```python
from build123d import *

# Parameters (mm, degrees)
SKETCH_1_W             = 36.9
SKETCH_1_H             = 36.9
EXTRUDE_1_DEPTH        = 20
SKETCH_2_R             = 4
CUT_EXTRUDE_1_DEPTH    = 36.9
SKETCH_3_R             = 6.5
CUT_EXTRUDE_2_DEPTH    = 3.5
CUT_EXTRUDE_3_DEPTH    = 51
FILLET_1_R             = 10
FILLET_2_R             = 5
SKETCH_5_W             = 16.9
SKETCH_5_H             = 16.9
SKETCH_5_W_2           = 7
SKETCH_5_H_2           = 7
CUT_EXTRUDE_4_DEPTH    = 16.55
HOLE_WIZARD_M3_1_D     = 2.5
HOLE_WIZARD_M3_1_DEPTH = 10
HOLE_WIZARD_M3_2_D     = 2.5
HOLE_WIZARD_M3_3_D     = 2.5
HOLE_WIZARD_M3_3_DEPTH = 10
FILLET_3_R             = 2
FILLET_7_R             = 2
CHAMFER_1_SIZE         = 0.3


with BuildPart() as part:
    # 草图1 → 凸台-拉伸1 (new, symmetric)
    with BuildSketch(Plane.XY):
        Rectangle(SKETCH_1_W, SKETCH_1_H)
    extrude(amount=EXTRUDE_1_DEPTH, both=True)

    # 草图2 → 切除-拉伸1 (cut)
    with BuildSketch(Plane(origin=(18.45, 0, 0), x_dir=(0, 0, -1), z_dir=(1, 0, 0))):
        with Locations((-11.25, -10)):
            Circle(SKETCH_2_R)
        Polygon((-1.5, 18.5), (-20, 0), (-20, 18.5), align=None)
    extrude(amount=-CUT_EXTRUDE_1_DEPTH, mode=Mode.SUBTRACT)

    # 草图3 → 切除-拉伸2 (cut)
    with BuildSketch(Plane(origin=(18.45, 0, 0), x_dir=(0, 0, -1), z_dir=(1, 0, 0))):
        with Locations((-11.25, -10)):
            Circle(SKETCH_3_R)
    cut_extrude_2 = extrude(amount=-CUT_EXTRUDE_2_DEPTH, mode=Mode.SUBTRACT)

    # 镜向1: 切除-拉伸2 across plane
    add(cut_extrude_2.mirror(Plane(origin=(0, 0, 0), x_dir=(0, 0, 1), z_dir=(1, 0, 0))), mode=Mode.SUBTRACT)

    # 草图4 → 切除-拉伸3 (cut)
    with BuildSketch(Plane(origin=(18.45, 0, 0), x_dir=(0, 0, -1), z_dir=(1, 0, 0))):
        Polygon((-20, 0), (-1.55, 0), (-1.55, 18.45), align=None)
    extrude(amount=-CUT_EXTRUDE_3_DEPTH, mode=Mode.SUBTRACT)

    # 圆角1
    fillet_1_edges = [part.edges().sort_by_distance(p)[0] for p in [
        (0, 0, 1.55),
    ]]
    fillet(fillet_1_edges, radius=FILLET_1_R)

    # 圆角2
    fillet_2_edges = [part.edges().sort_by_distance(p)[0] for p in [
        (0, -18.45, 20),
        (0, 0, 20),
    ]]
    fillet(fillet_2_edges, radius=FILLET_2_R)

    # 草图5 → 切除-拉伸4 (cut)
    with BuildSketch(Plane(origin=(0, 0, -20), x_dir=(-1, 0, 0), z_dir=(0, 0, -1))):
        Rectangle(SKETCH_5_W, SKETCH_5_H)
        with Locations((-11.95, 0)):
            Rectangle(SKETCH_5_W_2, SKETCH_5_H)
        with Locations((0, 11.95)):
            Rectangle(SKETCH_5_W, SKETCH_5_H_2)
        with Locations((11.95, 0)):
            Rectangle(SKETCH_5_W_2, SKETCH_5_H)
        with Locations((0, -11.95)):
            Rectangle(SKETCH_5_W, SKETCH_5_H_2)
    extrude(amount=-CUT_EXTRUDE_4_DEPTH, mode=Mode.SUBTRACT)

    # M3 螺纹孔1
    with Locations(Plane(origin=(0, 18.45, 0), x_dir=(1, 0, 0), z_dir=(0, 1, 0))):
        with Locations((-13.45, 10), (13.45, 10)):
            Hole(HOLE_WIZARD_M3_1_D / 2, depth=HOLE_WIZARD_M3_1_DEPTH)

    # M3 螺纹孔2 (through all)
    with Locations(Plane(origin=(18.45, 0, 0), x_dir=(0, 0, -1), z_dir=(1, 0, 0))):
        with Locations((10, -13.45)):
            hole_wizard_m3_2 = Hole(HOLE_WIZARD_M3_2_D / 2)

    # 镜向2: M3 螺纹孔2 across plane
    add(hole_wizard_m3_2.mirror(Plane(origin=(0, 0, 0), x_dir=(0, 0, 1), z_dir=(1, 0, 0))), mode=Mode.SUBTRACT)

    # M3 螺纹孔3
    with Locations(Plane(origin=(0, -18.45, 0), x_dir=(-1, 0, 0), z_dir=(0, -1, 0))):
        with Locations((10, 5), (-10, 5)):
            Hole(HOLE_WIZARD_M3_3_D / 2, depth=HOLE_WIZARD_M3_3_DEPTH)

    # 圆角3
    # the kernel refuses this fillet: 2 mm, written as the material it adds along each edge
    with BuildSketch(Plane(origin=(-15.45, 8.45, -20), x_dir=(1, 0, 0), z_dir=(0, 0, 1))) as fillet_3_piece_1_section:
        with BuildLine():
            CenterArc((FILLET_3_R, -FILLET_3_R), FILLET_3_R, 90, 90)
            Line((0, -FILLET_3_R), (0, 0))
            Line((0, 0), (FILLET_3_R, 0))
        make_face()
    fillet_3_piece_1 = extrude(amount=21.55, mode=Mode.PRIVATE)
    fillet_3_piece_1 = fillet_3_piece_1 - Plane(origin=(-13.45, 7.989094357, -10), x_dir=(-1, 0, 0), z_dir=(0, -1, 0)) * Cylinder(1.25, 52, mode=Mode.PRIVATE)
    add(fillet_3_piece_1)
    with BuildSketch(Plane(origin=(-15.45, -8.45, -20), x_dir=(0, 1, 0), z_dir=(0, 0, 1)), Plane(origin=(15.45, -8.45, -20), x_dir=(-1, 0, 0), z_dir=(0, 0, 1)), Plane(origin=(8.45, 15.45, -20), x_dir=(0, -1, 0), z_dir=(0, 0, 1)), Plane(origin=(-8.45, 15.45, -20), x_dir=(1, 0, 0), z_dir=(0, 0, 1))) as fillet_3_piece_2:
        with BuildLine():
            CenterArc((FILLET_3_R, -FILLET_3_R), FILLET_3_R, 90, 90)
            Line((0, -FILLET_3_R), (0, 0))
            Line((0, 0), (FILLET_3_R, 0))
        make_face()
    extrude(amount=21.55)
    with BuildSketch(Plane(origin=(-8.45, -15.45, -20), x_dir=(0, 1, 0), z_dir=(0, 0, 1))) as fillet_3_piece_3_section:
        with BuildLine():
            CenterArc((FILLET_3_R, -FILLET_3_R), FILLET_3_R, 90, 90)
            Line((0, -FILLET_3_R), (0, 0))
            Line((0, 0), (FILLET_3_R, 0))
        make_face()
    fillet_3_piece_3 = extrude(amount=21.55, mode=Mode.PRIVATE)
    fillet_3_piece_3 = fillet_3_piece_3 - Plane(origin=(-7.989094431, -13.45, -10), x_dir=(0, 0, 1), z_dir=(-1, 0, 0)) * Cylinder(1.25, 52, mode=Mode.PRIVATE)
    add(fillet_3_piece_3)
    with BuildSketch(Plane(origin=(8.45, -15.45, -20), x_dir=(-1, 0, 0), z_dir=(0, 0, 1))) as fillet_3_piece_4_section:
        with BuildLine():
            CenterArc((FILLET_3_R, -FILLET_3_R), FILLET_3_R, 90, 90)
            Line((0, -FILLET_3_R), (0, 0))
            Line((0, 0), (FILLET_3_R, 0))
        make_face()
    fillet_3_piece_4 = extrude(amount=21.55, mode=Mode.PRIVATE)
    fillet_3_piece_4 = fillet_3_piece_4 - Plane(origin=(7.989094875, -13.45, -10), x_dir=(0, 0, 1), z_dir=(-1, 0, 0)) * Cylinder(1.25, 52, mode=Mode.PRIVATE)
    add(fillet_3_piece_4)
    with BuildSketch(Plane(origin=(15.45, 8.45, -20), x_dir=(-1, 0, 0), z_dir=(0, 0, 1))) as fillet_3_piece_5_section:
        with BuildLine():
            CenterArc((FILLET_3_R, FILLET_3_R), FILLET_3_R, 180, 90)
            Line((0, FILLET_3_R), (0, 0))
            Line((0, 0), (FILLET_3_R, 0))
        make_face()
    fillet_3_piece_5 = extrude(amount=21.55, mode=Mode.PRIVATE)
    fillet_3_piece_5 = fillet_3_piece_5 - Plane(origin=(13.45, 7.989094431, -10), x_dir=(-1, 0, 0), z_dir=(0, -1, 0)) * Cylinder(1.25, 52, mode=Mode.PRIVATE)
    add(fillet_3_piece_5)
    # the kernel refuses this fillet: 2 mm, written as the material it takes off along each edge
    with BuildSketch(Plane(origin=(-8.45, 8.45, -25), x_dir=(-1, 0, 0), z_dir=(0, 0, 1)), Plane(origin=(8.45, -8.45, -25), x_dir=(1, 0, 0), z_dir=(0, 0, 1))) as fillet_3_2_piece_1:
        with BuildLine():
            CenterArc((FILLET_3_R, -FILLET_3_R), FILLET_3_R, 90, 90)
            Line((0, -FILLET_3_R), (0, 0))
            Line((0, 0), (FILLET_3_R, 0))
        make_face()
    extrude(amount=21.55, mode=Mode.SUBTRACT)
    with BuildSketch(Plane(origin=(-8.45, -8.45, -25), x_dir=(-1, 0, 0), z_dir=(0, 0, 1)), Plane(origin=(8.45, 8.45, -25), x_dir=(1, 0, 0), z_dir=(0, 0, 1))) as fillet_3_2_piece_2:
        with BuildLine():
            CenterArc((FILLET_3_R, FILLET_3_R), FILLET_3_R, 180, 90)
            Line((0, FILLET_3_R), (0, 0))
            Line((0, 0), (FILLET_3_R, 0))
        make_face()
    extrude(amount=21.55, mode=Mode.SUBTRACT)

    # 圆角7
    fillet_7_edges = [part.edges().sort_by_distance(p)[0] for p in [
        (0, 18.45, 1.55),
    ]]
    fillet(fillet_7_edges, radius=FILLET_7_R)

    # 镜向3: M3 螺纹孔2 across plane
    add(hole_wizard_m3_2.mirror(Plane.ZX), mode=Mode.SUBTRACT)

    # 倒角1
    chamfer_1_edges = [part.edges().sort_by_distance(p)[0] for p in [
        (18.45, -10, 17.75),
        (-18.45, -10, 17.75),
    ]]
    chamfer(chamfer_1_edges, length=CHAMFER_1_SIZE)


solid = part.part
```
Geometry check sheet. Reference: the model listing, model coordinates, mm. A direction names the side the tool comes from. Coordinates: 2 decimals unless noted, no trailing zeros. Order: outer loops, then holes, each group sorted by start corner. A loop starts at its lowest first (then second) coordinate and runs counter-clockwise, first axis right, second up. Notation, with made-up numbers: (29.5, 55.25) - (84.5, 55.25) arc R22 cw to (84.5, 88.25) - close; hole circle Ø2 at (56.25, -22). An arc over 180 degrees is marked (long way). Answer as a JSON object with one key per item and string values. Group by question number.
Item 1: Draft check along Y on faces 4 (the face through (-15.45, 0, -12)), 5 (the face through (0, 0, 13)), 6 (the face through (0, -9, 20)), 7 (the face through (-9.02, -9.05, -11.84)). Enter one of: +Y half, -Y half, draft (parallel to the pull), parting line (faces both ways), or undercut.
Item 2: Sectioned sample at C-C, the plane y = 1. Record the cut outline in (x, z), and give its area (3 significant figures).
Item 3: Tool access check on faces 1 (the face through (12.778, 16.471, -11.054)), 2 (the face through (-14.95, -7, 8)), 3 (the face through (-14.88, -7.85, -11.84)). Record the directions out of +Z, -Z, +X, -X, +Y, -Y that give a thin tool (end or side, any length) a straight path to the whole face; none if there is none.
Item 4: Depth check by flat-ended pin: pin 1 Ø1.7 at (x, z) = (6.5, 14) entering from +Y; pin 2 Ø5 at (x, y) = (-0.5, 2.5) entering from -Z; pin 3 Ø4 at (y, z) = (-13, 11.5) entering from +X. Enter the tip coordinate at first touch or a pass-through.
Item 5: Sectioned sample at B-B, the plane z = -12. Record the cut outline in (x, y).
Item 6: Sectioned sample at A-A, the plane x = 5.5. Record the cut outline in (y, z), and give its area (3 significant figures).
Item 7: Scan lines: probe 1 along Y at (x, z) = (12.25, -10); probe 2 along Z at (x, y) = (16, -13.45); probe 3 along Y at (x, z) = (5, -17.5). Record each from-to range of solid material in increasing order.
Resolved:
{
 "1": {"face 4": "undercut", "face 5": "+Y half", "face 6": "draft", "face 7": "undercut"},
 "2": {"outline": "(-18.45, -20) - (-15.45, -20) - (-15.45, -3.45) - (15.45, -3.45) - (15.45, -20) - (18.45, -20) - (18.45, 7.19) - (-18.45, 7.19) - close", "area": "492 mm^2"},
 "3": {"face 1": "+Y", "face 2": "-X", "face 3": "-Z"},
 "4": {"pin 1": "y = 0", "pin 2": "z = -3.45", "pin 3": "x = 14.95"},
 "5": {"outline": "(-18.45, -18.45) - (18.45, -18.45) - (18.45, 18.45) - (-18.45, 18.45) - close; hole (-15.45, -6.45) arc R2 ccw to (-13.45, -8.45) - (-10.45, -8.45) arc R2 cw to (-8.45, -10.45) - (-8.45, -13.45) arc R2 ccw to (-6.45, -15.45) - (6.45, -15.45) arc R2 ccw to (8.45, -13.45) - (8.45, -10.45) arc R2 cw to (10.45, -8.45) - (13.45, -8.45) arc R2 ccw to (15.45, -6.45) - (15.45, 6.45) arc R2 ccw to (13.45, 8.45) - (10.45, 8.45) arc R2 cw to (8.45, 10.45) - (8.45, 13.45) arc R2 ccw to (6.45, 15.45) - (-6.45, 15.45) arc R2 ccw to (-8.45, 13.45) - (-8.45, 10.45) arc R2 cw to (-10.45, 8.45) - (-13.45, 8.45) arc R2 ccw to (-15.45, 6.45) - close"},
 "6": {"outline": "(-18.45, -20) - (-15.45, -20) - (-15.45, -3.45) - (15.45, -3.45) - (15.45, -20) - (18.45, -20) - (18.45, -0.45) arc R2 ccw to (16.45, 1.55) - (10, 1.55) arc R10 cw to (0, 11.55) - (0, 15) arc R5 ccw to (-5, 20) - (-13.45, 20) arc R5 ccw to (-18.45, 15) - close; hole circle Ø8 at (-10, 11.25)", "area": "584 mm^2"},
 "7": {"probe 1": "-18.45 to -14.7, -12.2 to -8.45", "probe 2": "-20 to -11.25, -8.75 to 5.74, 16.76 to 20", "probe 3": "-18.45 to -15.45, 15.45 to 18.45"}
}
